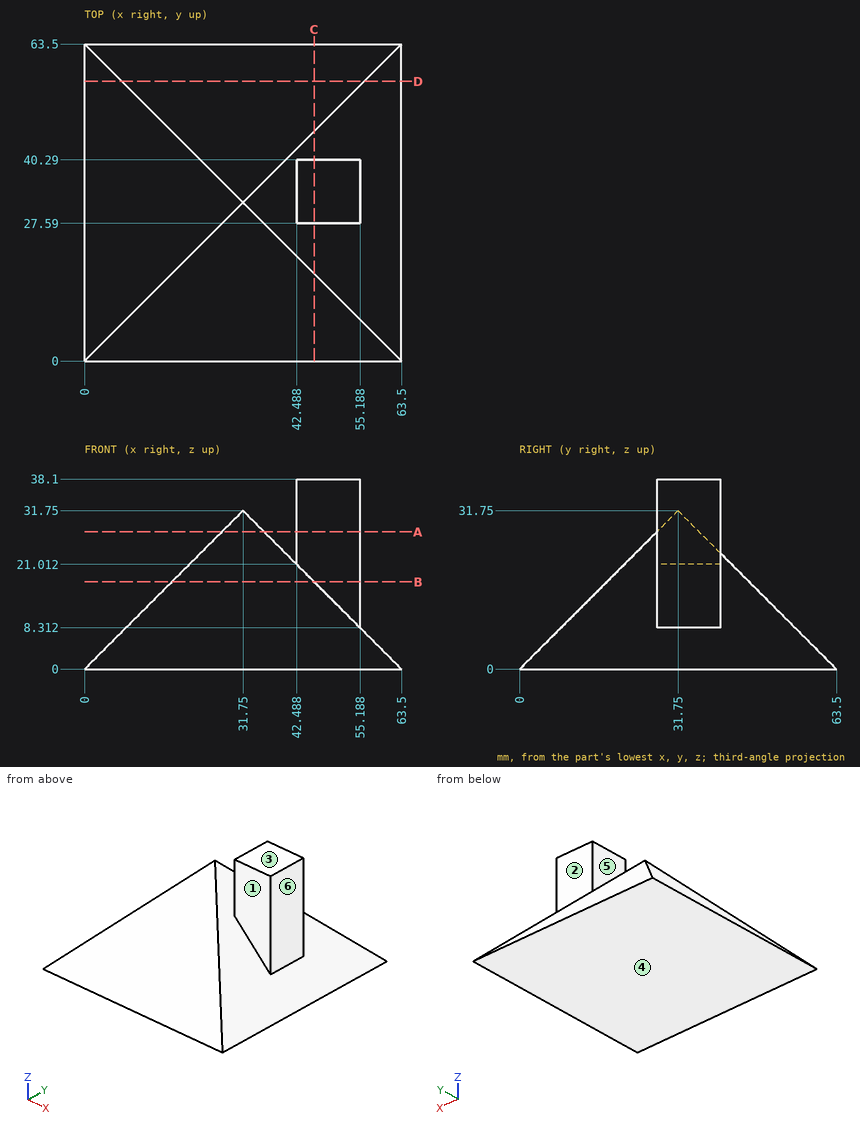
Study the drawing (mm; zero at the part's minimum x, y, z) and answer. A direction names the side the tool comes from. Round coordinates to 2 decimals unless told otherwise and drop trailing zeros. Order: outer loops, then holes, each group sorted by start corner. A loop starts at its lowest first (then second) coordinate and runs counter-clockwise, first axis right, second up. Notation, with made-up numbers: (-25, 3) - (9, 3) arc R35 ccw to (9, 36) - close; hole circle Ø7 at (0, 89). An arc over 180 degrees is marked (long way). Use one line per item in the form item = value. Start each with the question number.
(1) The part is cut by section B-B (z = 17.5). Give the vertices of the cut face in (x, y).
(2) Determine the mould class of the marked faces 4, 5 and 6 for opening direction X: +X half, -X half, draft (parallel to the pull), parting line (faces both ways), or undercut.
(3) For the marked faces 1, 2 and 3, determine the directions among +Z, -Z, +X, -X, +Y, -Y from which every point of the face is accessible in a straight line to the end or side of a thin tool.
(4) The part is cut by section D-D (y = 56). Give the vertices of the cut face in (x, z), then the cut area to 3 significant figures.
(5) The part is cut by section A-A (z = 27.5). Give the vertices of the cut face in (x, y).
(6) Flat-ended cylindrical pins translate along their axes: pin 1 Ø10 at (x, y) = (31.5, 38.5) entering from +Z; pin 2 Ø2 at (y, z) = (30, 17.5) entering from -X; pin 3 Ø6.5 at (y, z) = (35, 25.5) entering from -X. Find the tip coordinate at first contact, or state that the pin passes through.
(7) The part is cut by section C-C (x = 46). Give the vertices of the cut face in (y, z), then the cut area to 3 significant figures.
(8) Find the intervals of material crossed by line 1 along X through (y, z) = (30, 31); line 2 along Z through (x, y) = (40.5, 19); line 3 along Z through (x, y) = (17, 36), in increasing order. Write a range as from..to.
Checked values:
q1.outline = (17.5, 17.5) - (46, 17.5) - (46, 27.59) - (55.19, 27.59) - (55.19, 40.29) - (46, 40.29) - (46, 46) - (17.5, 46) - close
q2.face_4 = draft
q2.face_5 = undercut
q2.face_6 = +X half
q3.face_1 = +Z, +X, -Y
q3.face_2 = +Z, +X, +Y
q3.face_3 = +Z, +X, -X, +Y, -Y
q4.outline = (0, 0) - (63.5, 0) - (56, 7.5) - (7.5, 7.5) - close
q4.area = 420 mm^2
q5.outline = (27.5, 27.5) - (36, 27.5) - (36, 36) - (27.5, 36) - close; (42.49, 27.59) - (55.19, 27.59) - (55.19, 40.29) - (42.49, 40.29) - close
q6.pin_1 = 30
q6.pin_2 = 16.5
q6.pin_3 = 22.25
q7.outline = (0, 0) - (63.5, 0) - (46, 17.5) - (40.29, 17.5) - (40.29, 38.1) - (27.59, 38.1) - (27.59, 17.5) - (17.5, 17.5) - close
q7.area = 1,070 mm^2
q8.line_1 = 42.49..55.19
q8.line_2 = 0..19
q8.line_3 = 0..17
